```python
from build123d import *

# Parameters (mm, degrees)
SKETCH1_R           = 115.202561211
SKETCH1_R_2         = 64.402561211
BOSS_EXTRUDE1_DEPTH = 6.35
SKETCH2_R           = 20.32
BOSS_EXTRUDE2_DEPTH = 6.35


with BuildPart() as part:
    # Sketch1 → Boss-Extrude1 (new body)
    with BuildSketch(Plane(origin=(0, 0, 0), x_dir=(1, 0, 0), z_dir=(0, 1, 0))):
        Circle(SKETCH1_R)
        Circle(SKETCH1_R_2, mode=Mode.SUBTRACT)
    extrude(amount=BOSS_EXTRUDE1_DEPTH)

    # Sketch2 → Boss-Extrude2 (add)
    with BuildSketch(Plane(origin=(0, 6.35, 0), x_dir=(1, 0, 0), z_dir=(0, 1, 0))):
        with Locations((0, 64.402561211)):
            Circle(SKETCH2_R)
        with Locations((0, 115.202561211)):
            Circle(SKETCH2_R)
        with Locations((37.85487569, 52.102766501)):
            Circle(SKETCH2_R)
        with Locations((61.250475506, 19.901485895)):
            Circle(SKETCH2_R)
        with Locations((61.250475506, -19.901485895)):
            Circle(SKETCH2_R)
        with Locations((37.85487569, -52.102766501)):
            Circle(SKETCH2_R)
        with Locations((0, -64.402561211)):
            Circle(SKETCH2_R)
        with Locations((-37.85487569, -52.102766501)):
            Circle(SKETCH2_R)
        with Locations((-61.250475506, -19.901485895)):
            Circle(SKETCH2_R)
        with Locations((-61.250475506, 19.901485895)):
            Circle(SKETCH2_R)
        with Locations((-37.85487569, 52.102766501)):
            Circle(SKETCH2_R)
        with Locations((39.401596497, 108.254996665)):
            Circle(SKETCH2_R)
        with Locations((74.05077895, 88.250281849)):
            Circle(SKETCH2_R)
        with Locations((99.768344589, 57.601280605)):
            Circle(SKETCH2_R)
        with Locations((113.452375447, 20.004714817)):
            Circle(SKETCH2_R)
        with Locations((113.452375447, -20.004714817)):
            Circle(SKETCH2_R)
        with Locations((99.76834459, -57.601280605)):
            Circle(SKETCH2_R)
        with Locations((74.05077895, -88.250281849)):
            Circle(SKETCH2_R)
        with Locations((39.401596497, -108.254996665)):
            Circle(SKETCH2_R)
        with Locations((0, -115.202561211)):
            Circle(SKETCH2_R)
        with Locations((-39.401596497, -108.254996665)):
            Circle(SKETCH2_R)
        with Locations((-74.05077895, -88.250281849)):
            Circle(SKETCH2_R)
        with Locations((-99.768344589, -57.601280605)):
            Circle(SKETCH2_R)
        with Locations((-113.452375447, -20.004714817)):
            Circle(SKETCH2_R)
        with Locations((-113.452375447, 20.004714817)):
            Circle(SKETCH2_R)
        with Locations((-99.768344589, 57.601280605)):
            Circle(SKETCH2_R)
        with Locations((-74.05077895, 88.250281849)):
            Circle(SKETCH2_R)
        with Locations((-39.401596497, 108.254996665)):
            Circle(SKETCH2_R)
    extrude(amount=-BOSS_EXTRUDE2_DEPTH)


solid = part.part
```
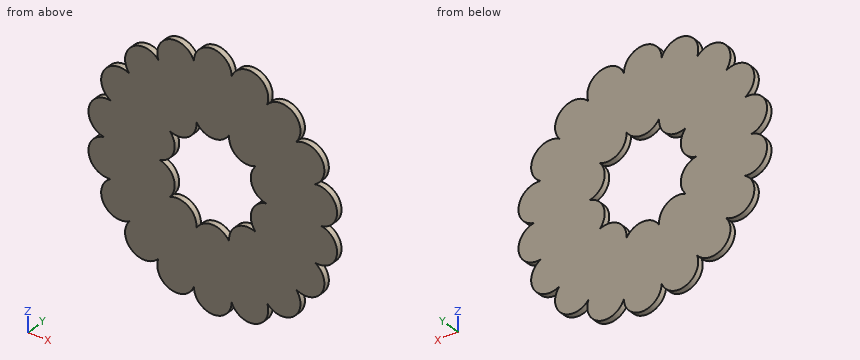
Can you work these out from the model? Positions are in its coordinate system, mm. Coordinates: 2 decimals unless noted, no trailing zeros. Loops run counter-clockwise (first coordinate to the right, second up) from the corner with the lowest first, then second, coordinate; pieces in that order, holes last. Notation, with made-up numbers: (7.5, 44) -> (18.5, 44) arc R27 ccw to (18.5, 75) -> close; hole circle Ø6 at (25.25, 1.5). An arc over 180 degrees is marked (long way). Answer as a JSON object with one key per item and string values.
1) Imagine slicing it at A-A (x = 0). Please give me the cut outline in (y, z), then the cut area to 3 significant figures.
Results:
{"outline": "(0, -135.52) -> (6.35, -135.52) -> (6.35, -44.08) -> (0, -44.08) -> close; (0, 44.08) -> (6.35, 44.08) -> (6.35, 135.52) -> (0, 135.52) -> close", "area": "1,160 mm^2"}
2) If I drill on line 1 (X direction, y = 0.5, z = -54); line 2 (X direction, y = 1, z = 103); line 3 (Z direction, x = 114, y = 5.25), over which ranges is the centre line in solid material (lowest first)?
Results:
{"line 1": "x = -119.77 to -17.62, -17.46 to 17.46, 17.62 to 119.77", "line 2": "x = -88.03 to -60.07, -59.03 to 59.03, 60.07 to 88.03", "line 3": "z = -72.11 to -43.1, -40.32 to 40.32, 43.1 to 72.11"}
3) For P1, Ø2, axis at x = 4.5, z = 46, coming from the -Y side; P2, Ø1, axis at y = 3.5, z = 27, coming from the -X side; P3, Ø2, axis at y = 2, z = -5.5, coming from the +X side; P4, Ø3, axis at y = 4, z = -57, coming from the +X side, each with a flat end and sliding along its axis, tell me the tip position at first contact or that it passes through.
Results:
{"P1": "stops at y = 0", "P2": "stops at x = -132.71", "P3": "stops at x = 128.64", "P4": "stops at x = 120.09"}
4) Imagine slicing it at B-B (z = -105). Please give me the cut outline in (x, y).
Results:
{"outline": "(-85.56, 0) -> (-62.55, 0) -> (-62.55, 6.35) -> (-85.56, 6.35) -> close; (-59.46, 0) -> (59.46, 0) -> (59.46, 6.35) -> (-59.46, 6.35) -> close; (62.55, 0) -> (85.56, 0) -> (85.56, 6.35) -> (62.55, 6.35) -> close"}
5) Imagine slicing it at C-C (x = 113.5). Please give me the cut outline in (y, z).
Results:
{"outline": "(0, -72.58) -> (6.35, -72.58) -> (6.35, -42.62) -> (0, -42.62) -> close; (0, -40.32) -> (6.35, -40.32) -> (6.35, 40.32) -> (0, 40.32) -> close; (0, 42.62) -> (6.35, 42.62) -> (6.35, 72.58) -> (0, 72.58) -> close"}
6) Imagine slicing it at D-D (y = 4). Please give me the cut outline in (x, z) (3 decimals).
Results:
{"outline": "(-117.018, 0) arc R20.32 ccw to (-109.961, -40.023) arc R20.32 ccw to (-89.641, -75.218) arc R20.32 ccw to (-58.509, -101.341) arc R20.32 ccw to (-20.32, -115.24) arc R20.32 ccw to (20.32, -115.24) arc R20.32 ccw to (58.509, -101.341) arc R20.32 ccw to (89.641, -75.218) arc R20.32 ccw to (109.961, -40.023) arc R20.32 ccw to (117.018, 0) arc R20.32 ccw to (109.961, 40.023) arc R20.32 ccw to (89.641, 75.218) arc R20.32 ccw to (58.509, 101.341) arc R20.32 ccw to (20.32, 115.24) arc R20.32 ccw to (-20.32, 115.24) arc R20.32 ccw to (-58.509, 101.341) arc R20.32 ccw to (-89.641, 75.218) arc R20.32 ccw to (-109.961, 40.023) arc R20.32 ccw to start; hole (-57.148, 0) arc R20.32 cw to (-46.233, -33.591) arc R20.32 cw to (-17.66, -54.351) arc R20.32 cw to (17.66, -54.351) arc R20.32 cw to (46.233, -33.591) arc R20.32 cw to (57.148, 0) arc R20.32 cw to (46.233, 33.591) arc R20.32 cw to (17.66, 54.351) arc R20.32 cw to (-17.66, 54.351) arc R20.32 cw to (-46.233, 33.591) arc R20.32 cw to start"}
